Source: CAD feature listing. Evaluate the final solid. Frame: model axes, mm. Face numbers are marked on the shaded views. Coordinates: 2 decimals unless noted, no trailing zeros.
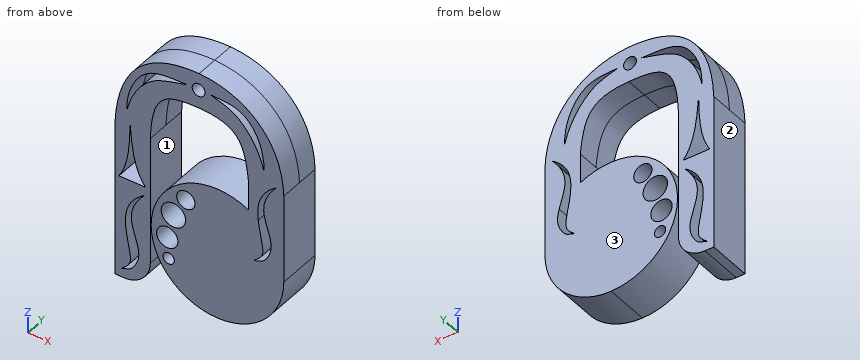
```python
from build123d import *

# Parameters (mm, degrees)
F1_DEPTH = 6.35
F2_R     = 7.62
F3_R     = 1.851317794
F3_R_2   = 2.623048948
F3_R_3   = 3.5099243314
F3_R_4   = 3.0648100187
F3_R_5   = 1.624839295
F4_DEPTH = 12.7


# Not quite as in the source:
# - a feature names something its author has since deleted; it is built from what else it names


with BuildPart() as f1:
    # F0 (on Front) → F1 (new body, symmetric)
    with BuildSketch(Plane.XZ):
        with BuildLine():
            Line((-47.4034676004, -12.1683157229), (-47.4034676004, -56.6183157229))
            Line((-47.4034676004, -56.6183157229), (-37.2434676004, -56.6183157229))
            Line((-37.2434676004, -56.6183157229), (-37.2434676004, -12.1683157229))
            add(Edge.make_bspline(
                [(-37.2434676004, -12.1683157229), (-36.7095838945, 1.4708520701), (-33.3203151822, 3.1873958426), (-22.9693437804, 3.0716842771)],
                knots=[0, 0, 0, 0, 20.8808096306, 20.8808096306, 20.8808096306, 20.8808096306], degree=3))
            add(Edge.make_bspline(
                [(-22.9693437804, 3.0716842771), (-11.9594718681, 2.6847659899), (-10.1360433424, -1.6166193699), (-9.0494676004, -12.1683158262)],
                knots=[0, 0, 0, 0, 20.6402654057, 20.6402654057, 20.6402654057, 20.6402654057], degree=3))
            Line((-9.0494676004, -12.1683158262), (-9.0494676004, -20.7198617879))
            ThreePointArc((-9.0494676004, -20.7198617879), (-7.6000300221, -21.5683616428), (-6.2309603269, -22.5412282663))
            add(Edge.make_bspline(
                [(-6.2309603269, -22.5412282663), (-6.2723652172, -22.1636683346), (-6.6533718861, -17.8378431816), (-5.6407446666, -13.777271871), (-0.9912915077, -10.6814840494)],
                knots=[0.5669230938, 0.5669230938, 0.5669230938, 0.5669230938, 0.6047158912, 1, 1, 1, 1], degree=3))
            add(Edge.make_bspline(
                [(-2.9873109532, -25.7642693151), (-3.3866343808, -24.3019783121), (-5.124946874, -19.6083809219), (-4.8990877844, -15.1703206189), (-0.9912915077, -10.6814840494)],
                knots=[0.5181753665, 0.5181753665, 0.5181753665, 0.5181753665, 0.6734400418, 1, 1, 1, 1], degree=3))
            ThreePointArc((-2.9873109532, -25.7642693151), (0.0569359866, -31.3207595659), (1.1105323996, -37.5683157229))
            Line((1.1105323996, -37.5683157229), (1.1105323996, -12.1683157229))
            add(Edge.make_bspline(
                [(1.1105323996, -12.1683157229), (0.5705629619, 4.0617453953), (-10.3604181223, 12.7446337565), (-23.2162306761, 13.2316842771)],
                knots=[0, 0, 0, 0, 35.1703198982, 35.1703198982, 35.1703198982, 35.1703198982], degree=3))
            add(Edge.make_bspline(
                [(-47.4034676004, -12.1683157229), (-46.5849920508, 7.3050484799), (-36.5418703402, 13.5184679613), (-23.2162306761, 13.2316842771)],
                knots=[0, 0, 0, 0, 35.0739565779, 35.0739565779, 35.0739565779, 35.0739565779], degree=3))
        make_face()
        with BuildLine():
            add(Edge.make_bspline(
                [(-45.5194190145, -54.1016533971), (-43.4073472429, -53.4859708194), (-42.3767122517, -53.0275311605), (-39.4416086551, -47.8736285865), (-43.2098006647, -39.8360561852), (-42.9273473132, -34.2859363798), (-39.0195510365, -29.7970998103)],
                knots=[0, 0, 0, 0, 0.1860018813, 0.3974429686, 0.6734400418, 1, 1, 1, 1], degree=3))
            add(Edge.make_bspline(
                [(-45.5194190145, -54.1016533971), (-43.4073472429, -52.4910938487), (-42.1962339672, -50.3443092376), (-45.4188846713, -39.9097980212), (-43.6690041954, -32.8928876319), (-39.0195510365, -29.7970998103)],
                knots=[0, 0, 0, 0, 0.2516171716, 0.6047158912, 1, 1, 1, 1], degree=3))
        make_face(mode=Mode.SUBTRACT)
        with BuildLine():
            add(Edge.make_bspline(
                [(-43.0450886488, -10.2955098264), (-43.0850870907, -18.8955254853), (-44.0450869501, -23.7755347043), (-46.2450906634, -27.1355397999)],
                knots=[0, 0, 0, 0, 17.1413716605, 17.1413716605, 17.1413716605, 17.1413716605], degree=3))
            add(Edge.make_bspline(
                [(-43.0450886488, -10.2955098264), (-42.4450859427, -18.8155258074), (-41.4850823581, -23.4555341303), (-38.685079664, -27.1355397999)],
                knots=[0, 0, 0, 0, 17.395294992, 17.395294992, 17.395294992, 17.395294992], degree=3))
            Line((-38.685079664, -27.1355397999), (-46.2450906634, -27.1355397999))
        make_face(mode=Mode.SUBTRACT)
        with BuildLine():
            add(Edge.make_bspline(
                [(-43.9962111413, -6.9482689141), (-42.8800281093, -1.4789610887), (-37.594435646, 6.055033296), (-32.2294885174, 6.9111710616), (-26.6296397895, 8.4384027869)],
                knots=[0, 0, 0, 0, 0.5184862256, 1, 1, 1, 1], degree=3))
            add(Edge.make_bspline(
                [(-43.9962111413, -6.9482689141), (-44.1630539416, -1.2757268376), (-39.7049183871, 8.2866771022), (-32.6861925423, 8.4215123206), (-26.6296397895, 8.4384027869)],
                knots=[0, 0, 0, 0, 0.513875061, 1, 1, 1, 1], degree=3))
        make_face(mode=Mode.SUBTRACT)
        with BuildLine():
            add(Edge.make_bspline(
                [(-19.9744962156, 8.4384027869), (-15.0681919771, 7.110938792), (-11.4060719241, 5.2750660976), (-6.2541036922, -1.0550173553), (-4.5138360001, -7.4359978316)],
                knots=[0, 0, 0, 0, 0.4513191083, 1, 1, 1, 1], degree=3))
            add(Edge.make_bspline(
                [(-19.9744962156, 8.4384027869), (-14.4520029301, 8.3067857058), (-9.1414830202, 7.6395398298), (-4.5325819981, -0.7140918586), (-4.5138360001, -7.4359978316)],
                knots=[0, 0, 0, 0, 0.4604709536, 1, 1, 1, 1], degree=3))
        make_face(mode=Mode.SUBTRACT)
        with BuildLine():
            ThreePointArc((-17.9394676004, -18.5183157229), (-31.409851782, -24.0979315413), (-36.9894676004, -37.5683157229))
            Line((-36.9894676004, -37.5683157229), (-17.9394676004, -37.5683157229))
            Line((-17.9394676004, -37.5683157229), (-17.9394676004, -18.5183157229))
        make_face()
        with BuildLine():
            ThreePointArc((-17.9394676004, -56.6183157229), (-4.4690834188, -51.0386999045), (1.1105323996, -37.5683157229))
            ThreePointArc((1.1105323996, -37.5683157229), (0.0569359866, -31.3207595659), (-2.9873109532, -25.7642693151))
            add(Edge.make_bspline(
                [(-7.4911594857, -34.9860376362), (-5.3790877141, -34.3703550585), (-4.3484527229, -33.9119153996), (-2.0900506569, -29.9462685874), (-2.6768006917, -26.9013334848), (-2.9873109532, -25.7642693151)],
                knots=[0, 0, 0, 0, 0.1860018813, 0.3974429686, 0.5181753665, 0.5181753665, 0.5181753665, 0.5181753665], degree=3))
            add(Edge.make_bspline(
                [(-7.4911594857, -34.9860376362), (-5.3790877141, -33.3754780878), (-4.243665121, -31.362860607), (-5.8855186547, -25.6912169104), (-6.2309603269, -22.5412282663)],
                knots=[0, 0, 0, 0, 0.2516171716, 0.5669230938, 0.5669230938, 0.5669230938, 0.5669230938], degree=3))
            ThreePointArc((-6.2309603269, -22.5412282663), (-7.6000300221, -21.5683616428), (-9.0494676004, -20.7198617879))
            ThreePointArc((-9.0494676004, -20.7198617879), (-13.3601962316, -19.0768913935), (-17.9394676004, -18.5183157229))
            Line((-17.9394676004, -18.5183157229), (-17.9394676004, -37.5683157229))
            Line((-17.9394676004, -37.5683157229), (-17.9394676004, -56.6183157229))
        make_face()
        with BuildLine():
            ThreePointArc((-36.9894676004, -37.5683157229), (-31.409851782, -51.0386999045), (-17.9394676004, -56.6183157229))
            Line((-17.9394676004, -56.6183157229), (-17.9394676004, -37.5683157229))
            Line((-17.9394676004, -37.5683157229), (-36.9894676004, -37.5683157229))
        make_face()
    extrude(amount=F1_DEPTH, both=True)

    # F2
    f2_edges = [f1.edges().sort_by_distance(p)[0] for p in [
        (-37.243468, 0, -56.618316),
    ]]
    fillet(f2_edges, radius=F2_R)

    # F3 (on Front) → F4 (cut, symmetric)
    with BuildSketch(Plane.XZ):
        with Locations((-23.3467891812, 8.3186188713)):
            Circle(F3_R)
        with Locations((-27.0257256925, -25.7905125618)):
            Circle(F3_R_2)
        with Locations((-30.5994562805, -31.8327024579)):
            Circle(F3_R_3)
        with Locations((-32.374959439, -39.1334928572)):
            Circle(F3_R_4)
        with Locations((-31.9626331329, -45.2065691352)):
            Circle(F3_R_5)
    extrude(amount=F4_DEPTH, both=True, mode=Mode.SUBTRACT)


solid = f1.part
```
1. Draft query along X for the marked faces 1, 2 and 3. Return one class per face: released by +X, released by -X, zero draft, split by the parting line, or undercut.
Findings:
face 1: undercut
face 2: released by -X
face 3: zero draft
2. Section query A-A on x = -15.5. Count the separate pieces of the cut face and the enclosed holes in it, plus the area to 3 significant figures.
Findings:
separate pieces: 3
enclosed holes: 0
area: 594 mm2
3. Ray query, line 1 (X direction, y = -1.5, z = -16.5); line 2 (Z direction, x = -17.5, y = 0.75); line 3 (X direction, y = 3.5, z = -47). Return the intervals inside material, ascending.
Findings:
line 1: x = -47.4 to -43.29, -42.44 to -37.24, -9.05 to -5.79, -4.39 to 1.11
line 2: z = -56.61 to -18.52, 2.38 to 7.72, 8.35 to 12.44
line 3: x = -47.4 to -43.35, -40.59 to -37.24, -34.49 to -1.39
4. Pin query (flat end, axial travel): P1, Ø8, axis at x = -32.37, z = -39.13, coming from the +Y side; P2, Ø3, axis at x = -23.35, z = 8.32, coming from the +Y side; P3, Ø1.5, axis at y = 2, z = -5, coming from the +X side; P4, Ø4, axis at x = -42.5, y = 0, coming from the +Z side. Return the tip coordinate at first contact, or that it passes through.
Findings:
P1: stops at y = 6.35
P2: passes through
P3: stops at x = 0.28
P4: stops at z = 7.46
